Geometry: final body of the model. Coordinates: model frame, mm. Coordinates: 2 decimals unless noted, no trailing zeros. Loops run counter-clockwise (first coordinate to the right, second up) from the corner with the lowest first, then second, coordinate; pieces in that order, holes last. Notation, with made-up numbers: M 74.25,-19 L 120.25,-19 A21 ccw 120.25,-7 Z; hole C 69.25,-13.5 d9. An arc over 180 degrees is marked long. Write each question's results on one line, items separated by ' | '. Start each with the question number.
from build123d import *

# Parameters (mm, degrees)
F0_R      = 10
F1_DEPTH  = 25
F1_FACE_R = 10
F2_DEPTH  = 25
F2_FACE_R = 10
F3_DEPTH  = 100


with BuildPart() as f1:
    # F0 (on Front) → F1 (new body)
    with BuildSketch(Plane.XZ):
        Circle(F0_R)
    extrude(amount=F1_DEPTH)

    # F1_face (on face) → F2 (join)
    with BuildSketch(Plane(origin=(0, 0, 0), x_dir=(1, 0, 0), z_dir=(0, 1, 0))):
        Circle(F1_FACE_R)
    extrude(amount=F2_DEPTH)

    # F2_face (on face) → F3 (join)
    with BuildSketch(Plane(origin=(0, 25, 0), x_dir=(1, 0, 0), z_dir=(0, 1, 0))):
        Circle(F2_FACE_R)
    extrude(amount=F3_DEPTH)


solid = f1.part
Item 1: Ray query, L1, parallel to X at y = -12.5, z = 0.25; L2, parallel to Z at x = -8.5, y = 63; L3, parallel to Z at x = 9, y = 56. Return the intervals inside material, ascending. Write a range as [from, to].
Item 2: Section A-A, the plane y = 28. Return loops of the section in (x, z).
Item 3: Section B-B, the plane z = -8. Return loops of the section in (x, y).
Item 4: Section C-C, the plane x = -8. Return loops of the section in (y, z), plus the area to 3 significant figures.
Item 5: Contact query for flat-ended pins moving along their axis: P1, Ø3, axis at x = 5, y = 49.5, coming from the -Z side; P2, Ø3, axis at x = -5, y = 62.5, coming from the +Z side; P3, Ø2, axis at y = 79.5, z = -3, coming from the -X side. Output: stop coordinate, or through.
Solutions:
1) L1: x = [-10, 10] | L2: z = [-5.27, 5.27] | L3: z = [-4.36, 4.36]
2) outline: C 0,0 d20
3) outline: M -6,-25 L 6,-25 L 6,125 L -6,125 Z
4) outline: M -25,-6 L 125,-6 L 125,6 L -25,6 Z | area: 1,800 mm²
5) P1: stops at z = -9.37 | P2: stops at z = 9.37 | P3: stops at x = -9.8
